from build123d import *

# Parameters (mm, degrees)
F1_DEPTH = 3


with BuildPart() as f1:
    # F0 (on Top) → F1 (new body)
    with BuildSketch(Plane.XY):
        with BuildLine():
            Line((1.25, -4), (1.25, -2.165064))
            ThreePointArc((1.25, -2.165064), (0, 2.5), (-1.25, -2.165064))
            Line((-1.25, -2.165064), (-1.25, -4))
            Line((-1.25, -4), (-3, -4))
            ThreePointArc((-3, -4), (-4.414214, -4.585786), (-5, -6))
            Line((-5, -6), (-5, -12))
            Line((-5, -12), (-4.65, -12))
            Line((-4.65, -12), (-4.65, -12.359054))
            ThreePointArc((-4.65, -12.359054), (-4.25, -13.406267), (-3.85, -12.359054))
            Line((-3.85, -12.359054), (-3.85, -12))
            Line((-3.85, -12), (-3.5, -12))
            Line((-3.5, -12), (-3.5, -6.2))
            ThreePointArc((-3.5, -6.2), (-3.441421, -6.058579), (-3.3, -6))
            Line((-3.3, -6), (-2.9, -6))
            ThreePointArc((-2.9, -6), (-2.758579, -6.058579), (-2.7, -6.2))
            Line((-2.7, -6.2), (-2.7, -24))
            Line((-2.7, -24), (-0.7, -24))
            Line((-0.7, -24), (-0.7, -17.5))
            ThreePointArc((-0.7, -17.5), (-0.553553, -17.146447), (-0.2, -17))
            Line((-0.2, -17), (0, -17))
            Line((0, -17), (0.2, -17))
            ThreePointArc((0.2, -17), (0.553553, -17.146447), (0.7, -17.5))
            Line((0.7, -17.5), (0.7, -24))
            Line((0.7, -24), (2.7, -24))
            Line((2.7, -24), (2.7, -6.2))
            ThreePointArc((2.7, -6.2), (2.758579, -6.058579), (2.9, -6))
            Line((2.9, -6), (3.3, -6))
            ThreePointArc((3.3, -6), (3.441421, -6.058579), (3.5, -6.2))
            Line((3.5, -6.2), (3.5, -12))
            Line((3.5, -12), (3.85, -12))
            Line((3.85, -12), (3.85, -12.359054))
            ThreePointArc((3.85, -12.359054), (4.25, -13.406267), (4.65, -12.359054))
            Line((4.65, -12.359054), (4.65, -12))
            Line((4.65, -12), (5, -12))
            Line((5, -12), (5, -6))
            ThreePointArc((5, -6), (4.414214, -4.585786), (3, -4))
            Line((3, -4), (1.25, -4))
        make_face()
    extrude(amount=F1_DEPTH)


solid = f1.part
For this review, take the finished solid that the model builds, in its own axes (mm). A direction names the side the tool comes from. Give positions to 0.01 mm unless a question says otherwise; leave off trailing zeros. Order: outer loops, then holes, each group sorted by start corner. A loop starts at its lowest first (then second) coordinate and runs counter-clockwise, first axis right, second up. Notation, with made-up numbers: M 28,52.25 L 50,52.25 A16 ccw 50,67.25 Z; hole C 23.25,72 d7. An arc over 180 degrees is marked long. Answer in a Markdown table with one row per item. Add a question column.
(1) Wall thickness on probe 1 along X at (y, z) = (-7.5, 1.3); probe 2 along X at (y, z) = (-21.5, 0.35); probe 3 along X at (y, z) = (-16.5, 2.4): over which ranges is each line inside the solid? List them lowest first. Write a range as [from, to].
(2) Consider section A-A on y = -18.5. State the section outline as (x, z) points, and give its area (3 significant figures).
(3) For pin 1 (1.5 mm diameter, centred on y = -21.5, z = 1, fed in from -X); pin 2 (0.6 mm diameter, centred on y = -3, z = 1.5, fed in from -X), all flat-tipped, find the tip position at first contact; note any pin that passes through.
(4) Consider section B-B on y = -7.5. State the section outline as (x, z) points, and give its area (3 significant figures).
(5) Consider section D-D on x = -4.25. State the section outline as (y, z) points, and give its area (3 significant figures).
(6) Consider section C-C on y = 0. State the section outline as (x, z) points.
(7) For faces 1 (the face through (3.5, -9, 1)), 2 (the face through (1.25, -3, 1)), 3 (the face through (-2, -4, 1)), list the 3-axis set-ups (+Z, -Z, +X, -X, +Y, -Y) from which the entire face can be reached by the end or side of a thin tool; tool diameter is ignored.
(8) Mouldability with a two-part tool opening along Y and no side actions: class faces 4 (the face through (-2, -24, 1)), 5 (the face through (-1.25, -3, 1)), 6 (the face through (-5, -9, 1)) as +Y half, -Y half, draft (parallel to the pull), parting line (faces both ways), or undercut.
Evaluation:
| question | item | result |
|---|---|---|
| 1 | probe 1 | x = [-5, -3.5], [-2.7, 2.7], [3.5, 5] |
| 1 | probe 2 | x = [-2.7, -0.7], [0.7, 2.7] |
| 1 | probe 3 | x = [-2.7, 2.7] |
| 2 | outline | M -2.7,0 L -0.7,0 L -0.7,3 L -2.7,3 Z; M 0.7,0 L 2.7,0 L 2.7,3 L 0.7,3 Z |
| 2 | area | 12.0 mm^2 |
| 3 | pin 1 | stops at x = -2.7 |
| 3 | pin 2 | stops at x = -1.25 |
| 4 | outline | M -5,0 L -3.5,0 L -3.5,3 L -5,3 Z; M -2.7,0 L 2.7,0 L 2.7,3 L -2.7,3 Z; M 3.5,0 L 5,0 L 5,3 L 3.5,3 Z |
| 4 | area | 25.2 mm^2 |
| 5 | outline | M -13.41,0 L -4.44,0 L -4.44,3 L -13.41,3 Z |
| 5 | area | 26.9 mm^2 |
| 6 | outline | M -2.5,0 L 2.5,0 L 2.5,3 L -2.5,3 Z |
| 7 | face 1 | +Z, -Z, -Y |
| 7 | face 2 | +Z, -Z, +X |
| 7 | face 3 | +Z, -Z, -X |
| 8 | face 4 | -Y half |
| 8 | face 5 | undercut |
| 8 | face 6 | draft |
